Can you work these out from the model? Positions are in its coordinate system, mm. A direction names the side the tool comes from. Give positions to 0.01 mm unless a question says otherwise; leave off trailing zeros. Order: outer loops, then holes, each group sorted by start corner. A loop starts at its lowest first (then second) coordinate and runs counter-clockwise, first axis right, second up. Notation, with made-up numbers: (32, 44.5) - (88, 44.5) arc R7 ccw to (88, 51.5) - close; hole circle Ø5 at (19, 71.5). An arc over 180 degrees is marked (long way). Answer as a JSON object with one key per item and string values.
```python
from build123d import *

# Parameters (mm, degrees)
SKETCH1_R           = 1.4605
BOSS_EXTRUDE1_DEPTH = 9.525
SKETCH2_W           = 17.145
SKETCH2_H           = 10.9474
CUT_EXTRUDE1_DEPTH  = 5


with BuildPart() as part:
    # Sketch1 → Boss-Extrude1 (new body)
    with BuildSketch(Plane(origin=(0, 0, 0), x_dir=(1, 0, 0), z_dir=(0, 1, 0))):
        with BuildLine():
            Line((0, 5.4737), (27.1526, 5.4737))
            ThreePointArc((27.1526, 5.4737), (32.6263, 0), (27.1526, -5.4737))
            Line((27.1526, -5.4737), (0, -5.4737))
            ThreePointArc((0, -5.4737), (-5.4737, 0), (0, 5.4737))
        make_face()
        with Locations(Location((0, 0, 0), (0, 0, 90))):
            Circle(SKETCH1_R, mode=Mode.SUBTRACT)
        with Locations(Location((27.1526, 0, 0), (0, 0, 90))):
            Circle(SKETCH1_R, mode=Mode.SUBTRACT)
    extrude(amount=BOSS_EXTRUDE1_DEPTH)

    # Sketch2 → Cut-Extrude1 (cut)
    with BuildSketch(Plane(origin=(0, 9.525, 0), x_dir=(1, 0, 0), z_dir=(0, 1, 0))):
        with Locations((13.5763, 0)):
            Rectangle(SKETCH2_W, SKETCH2_H)
    extrude(amount=-CUT_EXTRUDE1_DEPTH, mode=Mode.SUBTRACT)


solid = part.part
```
Q1. If we section it at B-B, the plane z = 0: Please give me the cut outline in (x, y) (1 decimal), then the cut area to 3 significant figures.
Recorded:
{"outline": "(-5.5, 0) - (-1.5, 0) - (-1.5, 9.5) - (-5.5, 9.5) - close; (1.5, 0) - (25.7, 0) - (25.7, 9.5) - (22.1, 9.5) - (22.1, 4.5) - (5, 4.5) - (5, 9.5) - (1.5, 9.5) - close; (28.6, 0) - (32.6, 0) - (32.6, 9.5) - (28.6, 9.5) - close", "area": "222 mm^2"}
Q2. Which directions (+Z, -Z, +X, -X, +Y, -Y) give clear straight access to the entire face, cutting with the end or side of a thin tool? Please do faces 1 (the face through (22.149, 7, 0)), 2 (the face through (1, 9.525, -1.3)).
Recorded:
{"face 1": "+Z, -Z, +Y", "face 2": "+Z, -Z, +X, -X, +Y"}
Q3. If we section it at D-D, the plane z = 2.25: Please give me the cut outline in (x, y) (3 decimals), then the cut area to 3 significant figures.
Recorded:
{"outline": "(-4.99, 0) - (32.142, 0) - (32.142, 9.525) - (22.149, 9.525) - (22.149, 4.525) - (5.004, 4.525) - (5.004, 9.525) - (-4.99, 9.525) - close", "area": "268 mm^2"}
Q4. We'd pull the mould along X, two halves only. Please class faces 3 (the face through (29, 9.525, 0)), 4 (the face through (5.004, 7, 0)), 5 (the face through (-5.472, 4.696, 0.12)), 6 (the face through (32.625, 4.696, -0.12)): released by +X, released by -X, zero draft, split by the parting line, or undercut.
Recorded:
{"face 3": "zero draft", "face 4": "undercut", "face 5": "released by -X", "face 6": "released by +X"}
Q5. If we section it at C-C, the plane y = 3: Please give me the cut outline in (x, z).
Recorded:
{"outline": "(0, -5.47) - (27.15, -5.47) arc R5.47 ccw to (27.15, 5.47) - (0, 5.47) arc R5.47 ccw to start; hole circle Ø2.92 at (0, 0); hole circle Ø2.92 at (27.15, 0)"}
Q6. I need wall thicknesses on L1, parallel to X at y = 2.5, z = 0; L2, parallel to Y at x = 14, z = -2.5 (3 decimals); L3, parallel to X at y = 6.75, z = 3.25. Which ranges of each line are inside material? Lowest first, please.
Recorded:
{"L1": "x = -5.47 to -1.46, 1.46 to 25.69, 28.61 to 32.63", "L2": "y = 0 to 4.525", "L3": "x = -4.4 to 5, 22.15 to 31.56"}
Q7. If we section it at A-A, the plane y = 7.75: Please give me the cut outline in (x, z), then the cut area to 3 significant figures.
Recorded:
{"outline": "(0, -5.47) - (5, -5.47) - (5, 5.47) - (0, 5.47) arc R5.47 ccw to start; (22.15, -5.47) - (27.15, -5.47) arc R5.47 ccw to (27.15, 5.47) - (22.15, 5.47) - close; hole circle Ø2.92 at (0, 0); hole circle Ø2.92 at (27.15, 0)", "area": "190 mm^2"}
Q8. I'm going to push flat-ended pins straight in: pin 1 Ø6 at (x, z) = (15.5, -2.5) entering from -Y; pin 2 Ø2 at (x, z) = (15, -3.5) entering from +Y (3 decimals); pin 3 Ø1.5 at (y, z) = (8, 1.5) entering from +X; pin 4 Ø1.5 at (y, z) = (7.5, -2.5) entering from -X. Where does each tip first touch, or does it pass through?
Recorded:
{"pin 1": "stops at y = 0", "pin 2": "stops at y = 4.525", "pin 3": "stops at x = 32.57", "pin 4": "stops at x = -5.19"}
